Check sheet for the modelled part. Datum: model origin and axes. Units: mm. A direction names the side the tool comes from. Give positions to 0.01 mm unless a question says otherwise; leave off trailing zeros. Write each loop counter-clockwise with the first axis right and the second up, starting at its lowest first coordinate (ties: lowest second). Pieces come first, ordered by that corner, then holes. Notation, with made-up numbers: M -23.5,-18.75 L 22.5,-18.75 A12 ccw 22.5,4.25 Z; hole C -14.5,55.25 d5. An arc over 180 degrees is marked long. One line per item, written item: value. Start each with the question number.
Autodesk Inventor part; units mm, degrees
ref_plane "YZ Plane" through (0, 0, 0) normal (1, 0, 0) x (0, 1, 0)
ref_plane "XZ Plane" through (0, 0, 0) normal (0, 1, 0) x (-1, 0, 0)
ref_plane "XY Plane" through (0, 0, 0) normal (0, 0, 1) x (1, 0, 0)
sketch "Skizze1" plane through (0, 0, 0) normal (0, 0, 1) x (1, 0, 0)
  line L0 (0, 0) -> (22.5, 0)
  line L1 (22.5, 0) -> (22.5, 75)
  line L2 (22.5, 75) -> (0, 75)
  line L3 (0, 75) -> (0, 0)
  line L4 (22.5, 80) -> (57.5, 80)
  line L5 (57.5, 80) -> (57.5, -80)
  line L6 (57.5, -80) -> (22.5, -80)
  line L7 (22.5, -80) -> (22.5, 80)
  line L8 (57.5, 0) -> (92.5, 0)
  line L9 (92.5, 0) -> (92.5, 35)
  line L10 (92.5, 35) -> (57.5, 35)
  line L11 (57.5, 35) -> (57.5, 0)
  line L12 (6, 75) -> (7.5, 75)
  line L13 (7.5, 75) -> (7.5, 73.5)
  line L14 (7.5, 73.5) -> (6, 73.5)
  line L15 (6, 73.5) -> (6, 75)
  dimension "d9" = 160
  dimension "d10" = 70
  dimension "d11" = 150
  dimension "d12" = 22.5
  dimension "d13" = 35
  dimension "d14" = 92.5
  dimension "d15" = 6
  dimension "d16" = 1.5
  dimension "d17" = 147
revolve "Umdrehung1" add sketch "Skizze1" angle 360 about axis through (0, 0, 0) along (1, 0, 0) contours L3 L2 L15 L14 L13 L1 L0 | L5 L10 L9 L8
extrude "Extrusion1" add sketch "Skizze1" along normal mid plane 160 contours L1 L7 L4 L5 L6
sketch "Skizze2" plane through (92.5, 0, 0) normal (1, 0, 0) x (0, 0, -1)
  circle A0 centre (0, 0) radius 35
hole "Bohrung1" at (92.5, 0, 0) direction (-1, 0, 0) diameter 50 end through all
sketch "Skizze3" plane through (57.5, -80, 80) normal (1, 0, 0) x (0, 0, -1)
  line L0 (0, 160) -> (160, 160)
  line L1 (0, 160) -> (30, 160)
  line L2 (30, 160) -> (30, 130)
  line L3 (30, 130) -> (0, 130)
  line L4 (0, 130) -> (0, 160)
  line L5 (145, 15) -> (15, 15)
  line L6 (15, 15) -> (15, 145)
  line L7 (15, 145) -> (145, 145)
  line L8 (145, 145) -> (145, 15)
  line L9 (145, 15) -> (15, 145) construction
  line L10 (15, 15) -> (145, 145) construction
  point P0 (80, 80)
  dimension "d28" = 30
  dimension "d29" = 30
  dimension "d30" = 130
  dimension "d31" = 130
hole "Bohrung2" at (57.5, 65, 65) direction (-1, 0, 0) diameter 10.5 end through all
pattern_circular "Runde Anordnung1" count 4 over 360 about axis through (75, 0, 0) along (1, 0, 0) of "Bohrung2"
sketch "Skizze5" plane through (0, 0, 0) normal (-1, 0, 0) x (0, 0, 1)
  line L0 (80, 80) -> (-80, 80)
  line L1 (-80, 80) -> (-80, -80)
  point P0 (0, 0)
  point P1 (-17.5, 50)
  point P2 (-80, 50)
  point P3 (-80, -50)
  dimension "d54" = 30
  dimension "d55" = 62.5
hole "Bohrung3" at (0, 50, -17.5) direction (1, 0, 0) diameter 8.5 depth 36 tip angle 118
sketch "Skizze6" plane through (22.5, 80, 80) normal (0, 1, 0) x (1, 0, 0)
  line L0 (35, 160) -> (35, 0)
  line L1 (5, 160) -> (35, 160)
  point P0 (-22.5, 80)
  point P1 (17.5, 97.5)
  point P2 (35, 130)
  point P3 (35, 30)
  dimension "d63" = 17.5
  dimension "d64" = 62.5
hole "Bohrung4" at (40, 80, -17.5) direction (0, -1, 0) diameter 8.376 depth 34.5 tip angle 118 counterbore diameter 20 counterbore depth 1.5
chamfer "Fase1" distance 2 angle 45 1 edges at (40, 78.5, -21.688)
chamfer "Fase2" distance 1 angle 45 8 edges at (0, -75, 0) (0, 0, 25) (92.5, 0, 25) (92.5, -35, 0) (57.5, 0, 80) (57.5, 80, 0) (57.5, 0, -80) (57.5, -80, 0)
fillet "Rundung2" radius 2 4 edges at (39.5, 80, -80) (39.5, 80, 80) (39.5, -80, -80) (39.5, -80, 80)
equation "\"d19\" = d9"
properties part number "Deckel_vorne" material "Stahl AISI 4130"
1) Cross-section at D-D (y = 65). State how many separate pieces and enclosed holes the cut face has, plus the area to 3 significant figures.
2) Cross-section at C-C (x = 15.5). Record the boundary of the cut face in (y, z).
3) Gauge pin test, flat ends, axial feed: pin 1 (9.5 mm diameter, centred on y = -65, z = 65, fed in from -X); pin 2 (3 mm diameter, centred on x = 11.5, y = 52, fed in from -Z); pin 3 (22 mm diameter, centred on x = 35.5, z = -13.5, fed in from +Y); pin 4 (12 mm diameter, centred on y = -10.5, z = -61.5, fed in from +X). Record the tip position at first contact, or that the pin passes through.
4) Tool access check on faces 1 (the flat face through (22.5, -24.1, -71.5)), 2 (the cylindrical face through (74, -28, 21)), 3 (the cylindrical face through (6.74, -15.933, 71.752)), 4 (the cylindrical face through (44.088, 60.783, -18.408)). Record the directions out of +Z, -Z, +X, -X, +Y, -Y that give a thin tool (end or side, any length) a straight path to the whole face; none if there is none.
5) Material ranges on L1, parallel to Z at x = 40, y = 69; L2, parallel to Y at x = 27, z = -63; L3, parallel to X at y = 79.45, z = -17.5, recorded low to high. Write a range as from..to.
6) Draft check along Z on faces 5 (the flat face through (92.5, -8, -25)), 6 (the cylindrical face through (3.465, -9.764, -74.362)), 7 (the conical face through (40.22, 43.42, -16.81)). Enter one of: released by +Z, released by -Z, zero draft, split by the parting line, or undercut.
Data:
1. separate pieces: 3
1. enclosed holes: 1
1. area: 6,480 mm2
2. outline: C 0,0 d150; hole C 0,0 d50; hole C 50,-17.5 d8.5
3. pin 1: passes through
3. pin 2: stops at z = -55.45
3. pin 3: stops at y = 80
3. pin 4: stops at x = 57.5
4. face 1: -X
4. face 2: +X
4. face 3: none
4. face 4: +Y
5. L1: z = -80..-68.4, -61.6..-21.69, -13.31..61.6, 68.4..80
5. L2: y = -80..-69.85, -60.15..60.15, 69.85..80
5. L3: x = 22.5..30, 50..57.05
6. face 5: zero draft
6. face 6: split by the parting line
6. face 7: undercut
